Here's how the part is built. I have some questions about the finished solid (model axes, mm). Face numbers are marked on the shaded views. A direction names the side the tool comes from. Give positions to 0.01 mm unless a question says otherwise; leave off trailing zeros. Order: outer loops, then holes, each group sorted by start corner. A loop starts at its lowest first (then second) coordinate and runs counter-clockwise, first axis right, second up. Notation, with made-up numbers: M 52,25.25 L 58,25.25 A10 ccw 58,44.25 Z; hole C 15.25,18 d11. An arc over 180 degrees is marked long. Use one line per item in the form item = value.
from build123d import *

# Parameters (mm, degrees)
F0_W     = 175
F0_H     = 105
F1_DEPTH = 10
F2_DEPTH = 42
F3_W     = 182.5
F3_H     = 15
F4_DEPTH = 7.5


with BuildPart() as f1:
    # F0 (on Front) → F1 (new body)
    with BuildSketch(Plane.XZ):
        Rectangle(F0_W, F0_H)
    extrude(amount=F1_DEPTH)

    # F0 (on Front) → F2 (join)
    with BuildSketch(Plane.XZ):
        Polygon((-87.5, 52.5), (87.5, 52.5), (87.5, 60), (-95, 60), (-95, -60), (87.5, -60), (87.5, -52.5), (-87.5, -52.5), align=None)
    extrude(amount=F2_DEPTH)

    # F3 (on face) → F4 (join)
    with BuildSketch(Plane.XZ.offset(42)):
        with Locations((-3.75, 67.5)):
            Rectangle(F3_W, F3_H)
        with Locations((-3.75, -67.5)):
            Rectangle(F3_W, F3_H)
    extrude(amount=-F4_DEPTH)


solid = f1.part
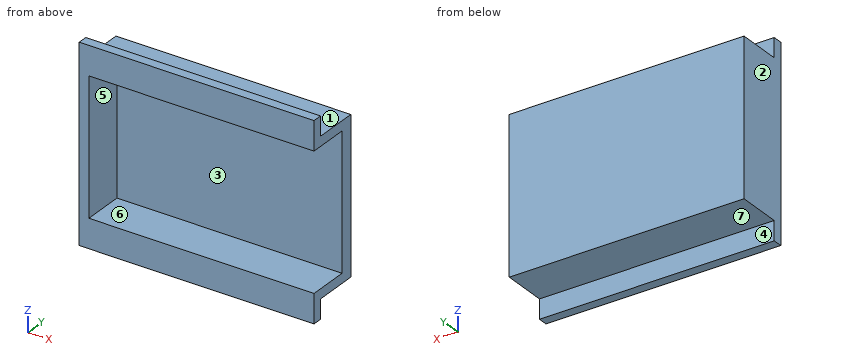
Q1. I want a section at B-B on x = 40. Write out the boundary of the cut face in (y, z).
Found:
outline = M -42,-75 L -34.5,-75 L -34.5,-60 L 0,-60 L 0,60 L -34.5,60 L -34.5,75 L -42,75 L -42,52.5 L -10,52.5 L -10,-52.5 L -42,-52.5 Z
Q2. I want a section at D-D on y = -38.5. Write out the boundary of the cut face in (x, z), then the cut area to 3 significant figures.
Found:
outline = M -95,-75 L 87.5,-75 L 87.5,-52.5 L -87.5,-52.5 L -87.5,52.5 L 87.5,52.5 L 87.5,75 L -95,75 Z
area = 9,000 mm²
Q3. I'm going to push flat-ended pins straight in: pin 1 Ø16 at (x, y) = (28, -26) entering from +Z; pin 2 Ø8 at (x, y) = (33.5, -21) entering from -Z; pin 3 Ø12 at (x, z) = (37, 70.5) entering from +Y. Where does each tip first touch, or does it pass through?
Found:
pin_1 = 60
pin_2 = -60
pin_3 = -34.5
Q4. Thinking about a two-plate mould opening in Z: for the marked faces 4, 5, 6 and 7, which applies, +Z half, -Z half, draft (parallel to the pull), parting line (faces both ways), or undercut?
Found:
face_4 = draft
face_5 = undercut
face_6 = undercut
face_7 = -Z half
Q5. I need wall thicknesses on L1, parallel to Z at x = -70.5, y = -20.5; L2, parallel to Z at x = 2, y = -38; L3, parallel to Y at x = -48.5, z = -22. Which ranges of each line are inside material? Lowest first, please.
Found:
L1 = -60 to -52.5, 52.5 to 60
L2 = -75 to -52.5, 52.5 to 75
L3 = -10 to 0
Q6. I want a section at A-A on y = -30. Write out the boundary of the cut face in (x, z), then the cut area to 4 significant figures.
Found:
outline = M -95,-60 L 87.5,-60 L 87.5,-52.5 L -87.5,-52.5 L -87.5,52.5 L 87.5,52.5 L 87.5,60 L -95,60 Z
area = 3,525 mm²
Q7. I want a section at C-C on z = 34. Write out the boundary of the cut face in (x, y).
Found:
outline = M -95,-42 L -87.5,-42 L -87.5,-10 L 87.5,-10 L 87.5,0 L -95,0 Z
Q8. On a 3-axis mill with a long thin cutter (end or side, diameter ignored), from which of +Z, -Z, +X, -X, +Y, -Y can I reach the whole of each face in a straight line? I mean the marked faces 1, 2 and 3. Say none if no direction works.
Found:
face_1 = +Z, +X, -X, +Y
face_2 = +Z, -Z, -X, +Y, -Y
face_3 = +X, -Y
